The model under review builds one solid part; all positions refer to its coordinate system, in mm. A direction names the side the tool comes from. Give positions to 0.01 mm unless a question says otherwise; leave off trailing zeros. Write each loop counter-clockwise with the first axis right and the second up, starting at its lowest first coordinate (ties: lowest second). Pieces come first, ordered by that corner, then holes. Notation, with made-up numbers: M 31.25,51 L 49.25,51 A17 ccw 49.25,69 Z; hole C -34,-17.75 d3. An arc over 180 degrees is marked long. Write item = value, one per line. Start each with the question number.
```python
from build123d import *

# Parameters (mm, degrees)
F1_DEPTH = 76.2
F3_DEPTH = 31.751


with BuildPart() as f1:
    # F0 (on Right) → F1 (new body)
    with BuildSketch(Plane.YZ):
        Polygon((15.875, 15.875), (-15.875, 15.875), (-15.875, -15.875), (-0.79375, -15.875), (-0.79375, 1.397), (0.79375, 1.397), (0.79375, -15.875), (15.875, -15.875), align=None)
    extrude(amount=F1_DEPTH)

    # F2 (on face) → F3 (cut, through all)
    with BuildSketch(Plane.XZ.offset(15.875)):
        Polygon((76.2, -15.875), (76.2, 15.875), (44.45, -15.875), align=None)
    extrude(amount=-F3_DEPTH, mode=Mode.SUBTRACT)


solid = f1.part
```
Item 1: We need section D-D, the plane y = -7.5. Write out the cut boundary in (x, z) (3 decimals).
Item 2: Clearance check with a flat-ended pin moving along its axis: P1, Ø1.3, axis at x = 17, y = 0, coming from the -Z side. State where the tip first meets the part, or that it passes through.
Item 3: We need section A-A, the plane z = -9.5. Write out the cut boundary in (x, y) (3 decimals).
Item 4: We need section B-B, the plane x = 14. Write out the cut boundary in (y, z) (3 decimals), and give its area (3 significant figures).
Item 5: For faces 1 (the flat face through (30, 0, 1.397)), 2 (the flat face through (60.547, -3.75, 0.222)), list the 3-axis set-ups (+Z, -Z, +X, -X, +Y, -Y) from which the entire face can be reached by the end or side of a thin tool; tool diameter is ignored.
Item 6: The part is to be moulded in two halves that separate along Y. For faces 3 (the flat face through (22, 8, -15.875)), 4 (the flat face through (29, -15.875, 0)), 5 (the flat face through (24, -0.794, -7)), say which applies: released by +Y, released by -Y, zero draft, split by the parting line, or undercut.
Item 7: We need section C-C, the plane z = -1.5. Write out the cut boundary in (x, y) (3 decimals).
Item 8: To check wall thickness, follow probe 1 along Y at (x, z) = (26, -3.5) (3 decimals); probe 2 along Z at (x, y) = (20.5, -0.5) (3 decimals); probe 3 along X at (y, z) = (11, -8) (3 decimals). State the ranges of each line that lie inside material, in increasing order. Write a range as [from, to].
Worked out:
q1.outline = M 0,-15.875 L 44.45,-15.875 L 76.2,15.875 L 0,15.875 Z
q2.P1 = 1.4
q3.outline = M 0,-15.875 L 50.825,-15.875 L 50.825,-0.794 L 0,-0.794 Z; M 0,0.794 L 50.825,0.794 L 50.825,15.875 L 0,15.875 Z
q4.outline = M -15.875,-15.875 L -0.794,-15.875 L -0.794,1.397 L 0.794,1.397 L 0.794,-15.875 L 15.875,-15.875 L 15.875,15.875 L -15.875,15.875 Z
q4.area = 981 mm²
q5.face_1 = -Z, +X, -X
q5.face_2 = -Z, +X, +Y, -Y
q6.face_3 = zero draft
q6.face_4 = released by -Y
q6.face_5 = undercut
q7.outline = M 0,-15.875 L 58.825,-15.875 L 58.825,-0.794 L 0,-0.794 Z; M 0,0.794 L 58.825,0.794 L 58.825,15.875 L 0,15.875 Z
q8.probe_1 = [-15.875, -0.794], [0.794, 15.875]
q8.probe_2 = [1.397, 15.875]
q8.probe_3 = [0, 52.325]
